CAD build for the part. Positions are in the model's coordinates, mm. Round coordinates to 2 decimals unless told otherwise and drop trailing zeros. Loops run counter-clockwise (first coordinate to the right, second up) from the corner with the lowest first, then second, coordinate; pieces in that order, holes last.
from build123d import *

# Parameters (mm, degrees)
EXTRUDE_1_DEPTH       = 244
EXTRUDE_3_DEPTH       = 244
PATTERN_CURVE_1_COUNT = 11
PATTERN_CURVE_1_PITCH = 10
SKETCH_3_R            = 2.25
CUT_EXTRUDE_1_DEPTH   = 6
SKETCH_4_R            = 1.6
CUT_EXTRUDE_2_DEPTH   = 6


with BuildPart() as part:
    # Эскиз1 → Вытянуть1 (new body)
    with BuildSketch(Plane.XY):
        with BuildLine():
            Line((0, 40), (1.528979332, 40))
            ThreePointArc((1.528979332, 40), (2.225614441, 39.717425624), (2.528547087, 39.029399052))
            Line((2.528547087, 39.029399052), (3.5, 6))
            Line((3.5, 6), (118.5, 6))
            Line((118.5, 6), (119.471452913, 39.029399052))
            ThreePointArc((119.471452913, 39.029399052), (119.774385559, 39.717425624), (120.471020668, 40))
            Line((120.471020668, 40), (122, 40))
            Line((122, 40), (122, 0))
            Line((122, 0), (0, 0))
            Line((0, 0), (0, 40))
        make_face()
    extrude(amount=EXTRUDE_1_DEPTH)

    # Эскиз2 → Вытянуть3 (add)
    with BuildSketch(Plane.XY.offset(244)):
        with BuildLine():
            Line((10.5, 39.5), (9.25, 6))
            Line((9.25, 6), (12.75, 6))
            Line((12.75, 6), (11.5, 39.5))
            ThreePointArc((11.5, 39.5), (11, 40), (10.5, 39.5))
        make_face()
    extrude_3 = extrude(amount=-EXTRUDE_3_DEPTH)

    # Кривая1: Вытянуть3 ×11
    with Locations(*[(i * PATTERN_CURVE_1_PITCH, 0, 0) for i in range(1, PATTERN_CURVE_1_COUNT)]):
        add(extrude_3)

    # Эскиз3 → Вырез-Вытянуть1 (cut)
    with BuildSketch(Plane.XZ):
        with Locations((26, 236)):
            Circle(SKETCH_3_R)
        with Locations((96, 236)):
            Circle(SKETCH_3_R)
        with Locations(Location((96, 8, 0), (0, 0, 180))):
            Circle(SKETCH_3_R)
        with Locations(Location((26, 8, 0), (0, 0, 180))):
            Circle(SKETCH_3_R)
    extrude(amount=-CUT_EXTRUDE_1_DEPTH, mode=Mode.SUBTRACT)

    # Эскиз4 → Вырез-Вытянуть2 (cut)
    with BuildSketch(Plane(origin=(147.933613103, 0, 237.946321054), x_dir=(-1, 0, 0), z_dir=(0, -1, 0))):
        with Locations(Location((42.433613103, 130.446321054, 0), (0, 0, 180))):
            Circle(SKETCH_4_R)
        with Locations(Location((85.933613103, 217.946321054, 0), (0, 0, 180))):
            Circle(SKETCH_4_R)
        with Locations(Location((85.933613103, 82.946321054, 0), (0, 0, 180))):
            Circle(SKETCH_4_R)
    extrude(amount=-CUT_EXTRUDE_2_DEPTH, mode=Mode.SUBTRACT)


solid = part.part
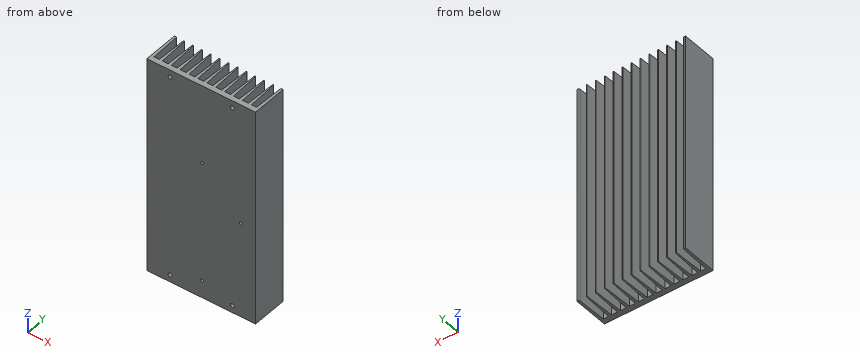
Item 1: Flat gauge pins, fed straight in: P1, Ø5, axis at x = 26.5, z = 138.5, coming from the +Y side; P2, Ø1.9, axis at x = 62, z = 155.5, coming from the -Y side. Where does each tip first touch, or does it go through?
Verdict:
P1: stops at y = 6
P2: stops at y = 6
Item 2: Cut at B-B (z = 236). State how many separate pieces and enclosed holes the cut face has, plus the area to 3 significant figures.
Verdict:
separate pieces: 3
enclosed holes: 0
area: 1,720 mm2
Item 3: Cut at A-A (x = 96). List the corners of the cut face in (y, z), plus the area to 3 significant figures.
Verdict:
outline: (0, 0) - (6, 0) - (6, 5.75) - (0, 5.75) - close; (0, 10.25) - (6, 10.25) - (6, 233.75) - (0, 233.75) - close; (0, 238.25) - (6, 238.25) - (6, 244) - (0, 244) - close
area: 1,410 mm2
Item 4: Wall check: L1, parallel to Z at x = 96, y = 4.7; L2, parallel to X at y = 1.9, z = 155; L3, parallel to Z at x = 105.5, y = 2.45. Give the ranges that are in metal, low to high.
Verdict:
L1: z = 0 to 5.75, 10.25 to 233.75, 238.25 to 244
L2: x = 0 to 60.4, 63.6 to 122
L3: z = 0 to 105.9, 109.1 to 244
